```python
from build123d import *

# Parameters (mm, degrees)
SALIENTE_EXTRUIR1_DEPTH = 11.8
CROQUIS7_R              = 5.525
CROQUIS7_R_2            = 2.45
SALIENTE_EXTRUIR2_DEPTH = 4.3
SALIENTE_EXTRUIR4_DEPTH = 2.5


with BuildPart() as part:
    # Croquis3 → Saliente-Extruir1 (new body)
    with BuildSketch(Plane(origin=(0, 0, 0), x_dir=(1, 0, 0), z_dir=(0, 1, 0))):
        Polygon((-11.35, 11.25), (11.35, 11.25), (11.35, 6.95), (16.35, 6.95), (16.35, 4.45), (11.35, 4.45), (11.35, -11.25), (-11.35, -11.25), (-11.35, 4.45), (-16.35, 4.45), (-16.35, 6.95), (-11.35, 6.95), align=None)
    extrude(amount=SALIENTE_EXTRUIR1_DEPTH)

    # Croquis7 → Saliente-Extruir2 (add)
    with BuildSketch(Plane(origin=(0, 0, -11.25), x_dir=(-1, 0, 0), z_dir=(0, 0, -1))):
        with Locations((5.825, 5.9)):
            Circle(CROQUIS7_R)
        with Locations((0, 5.9)):
            Circle(CROQUIS7_R_2)
    extrude(amount=SALIENTE_EXTRUIR2_DEPTH)

    # Croquis8 → Saliente-Extruir4 (add)
    with BuildSketch(Plane(origin=(0, 0, -15.55), x_dir=(-1, 0, 0), z_dir=(0, 0, -1))):
        with BuildLine():
            ThreePointArc((8.225, 5.9), (7.522056275, 7.597056275), (5.825, 8.3))
            Line((5.825, 8.3), (5.825, 6.475))
            ThreePointArc((5.825, 6.475), (6.231586399, 6.306586399), (6.4, 5.9))
            ThreePointArc((6.4, 5.9), (6.231586399, 5.493413601), (5.825, 5.325))
            Line((5.825, 5.325), (5.825, 3.5))
            ThreePointArc((5.825, 3.5), (7.522056275, 4.202943725), (8.225, 5.9))
        make_face()
        with BuildLine():
            Line((5.825, 6.475), (5.825, 8.3))
            ThreePointArc((5.825, 8.3), (3.425, 5.9), (5.825, 3.5))
            Line((5.825, 3.5), (5.825, 5.325))
            ThreePointArc((5.825, 5.325), (5.25, 5.9), (5.825, 6.475))
        make_face()
    extrude(amount=SALIENTE_EXTRUIR4_DEPTH)


solid = part.part
```
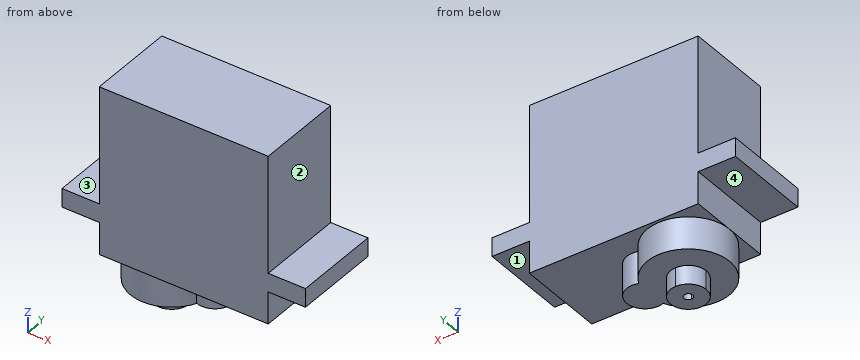
Geometry: final body of the model. Coordinates: model frame, mm. Face numbers are marked on the shaded views. A direction names the side the tool comes from. Coordinates: 2 decimals unless noted, no trailing zeros. Order: outer loops, then holes, each group sorted by start corner. A loop starts at its lowest first (then second) coordinate and runs counter-clockwise, first axis right, second up. Notation, with made-up numbers: (-4.5, -20.5) - (0.5, -20.5) arc R22 cw to (0.5, -13.5) - close; hole circle Ø7 at (-34.75, 17.25). An arc over 180 degrees is marked (long way). Return JSON: item names as keys, results as strings. Group by question number.
1. Set-up query: the marked faces 1, 2, 3 and 4. Return all of +Z, -Z, +X, -X, +Y, -Y with unobstructed straight access to the full face (end or side cutting, diameter ignored); none if empty.
2. Pin query (flat end, axial travel): pin 1 (3 mm diameter, centred on y = 1.5, z = 4.5, fed in from -X); pin 2 (2 mm diameter, centred on y = 5, z = -8.5, fed in from -X); pin 3 (3 mm diameter, centred on y = 8.5, z = -13.5, fed in from +X). Return the tip coordinate at first contact, or that it passes through.
3. Cut plane A-A (x = 0). Output: boundary loops of the cut face in (y, z), plus the area to 3 significant figures.
4. Cut plane C-C (z = 5). Output: boundary loops of the cut face in (x, y).
5. Cut plane B-B (y = 8.75). Output: boundary loops of the cut face in (x, z), plus the area to 3 significant figures.
6. Cut plane D-D (x = -10). Output: boundary loops of the cut face in (y, z).
7. Material intervals for line 1 along Z through (x, y) = (-13.5, 10); line 2 along Z through (x, y) = (0, 7); line 3 along X through (y, z) = (6.25, -1.5), sorted ascending. Write a range as [from, to].
Resolved:
{
 "1": {"face 1": "-Z, +X, +Y, -Y", "face 2": "+Z, +X, +Y, -Y", "face 3": "+Z, -X, +Y, -Y", "face 4": "-Z, -X, +Y, -Y"},
 "2": {"pin 1": "stops at x = -11.35", "pin 2": "stops at x = -11.35", "pin 3": "stops at x = 2.19"},
 "3": {"outline": "(0, -11.25) - (3.45, -11.25) - (3.45, -15.55) - (8.35, -15.55) - (8.35, -11.25) - (11.8, -11.25) - (11.8, 11.25) - (0, 11.25) - close", "area": "287 mm²"},
 "4": {"outline": "(-11.35, 0) - (11.35, 0) - (11.35, 11.8) - (-11.35, 11.8) - close"},
 "5": {"outline": "(-16.35, -6.95) - (-11.35, -6.95) - (-11.35, -11.25) - (-10.56, -11.25) - (-10.56, -15.55) - (-1.09, -15.55) - (-1.09, -11.25) - (11.35, -11.25) - (11.35, -6.95) - (16.35, -6.95) - (16.35, -4.45) - (11.35, -4.45) - (11.35, 11.25) - (-11.35, 11.25) - (-11.35, -4.45) - (-16.35, -4.45) - close", "area": "576 mm²"},
 "6": {"outline": "(0, -11.25) - (2.28, -11.25) - (2.28, -15.55) - (9.52, -15.55) - (9.52, -11.25) - (11.8, -11.25) - (11.8, 11.25) - (0, 11.25) - close"},
 "7": {"line 1": "z = [-6.95, -4.45]", "line 2": "z = [-15.55, 11.25]", "line 3": "x = [-11.35, 11.35]"}
}
